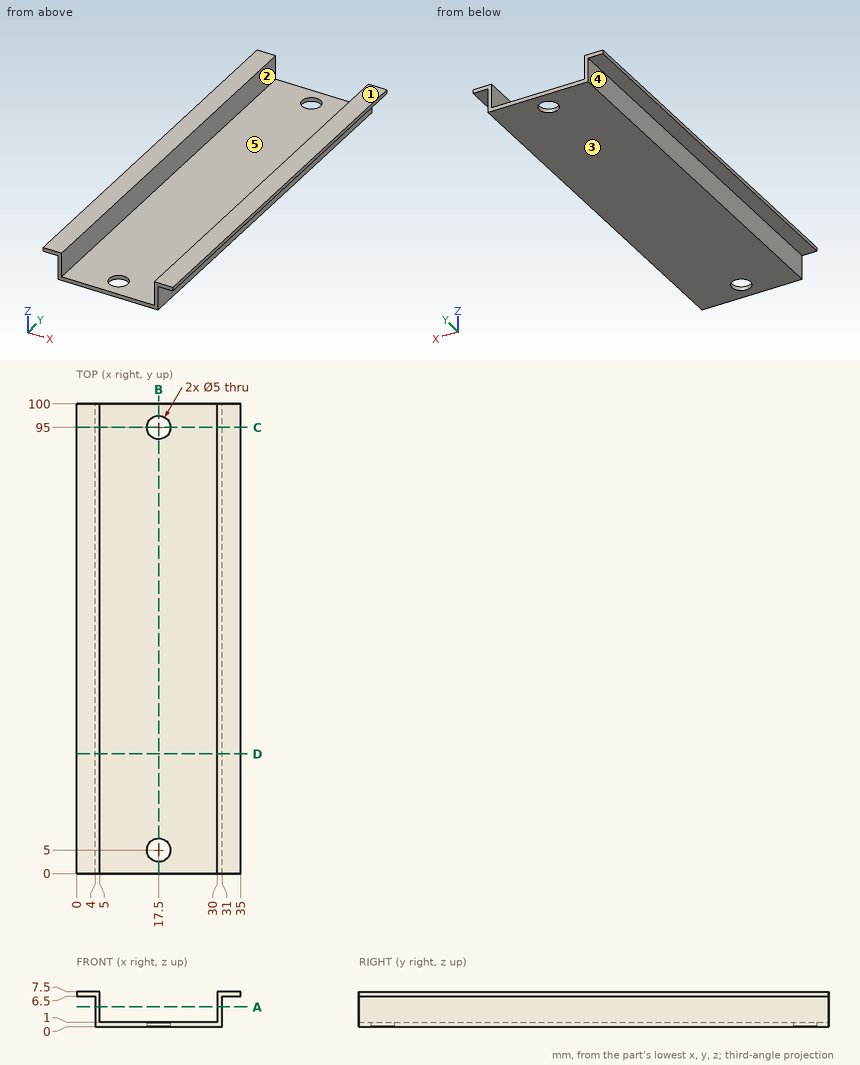
Verification items for this drawing (mm, ordinates from the low corner). A direction names the side the tool comes from. Give positions to 0.01 mm unless a question says otherwise; leave off trailing zeros. Loops run counter-clockwise (first coordinate to the right, second up) from the corner with the lowest first, then second, coordinate; pieces in that order, holes last.
1. Cross-section at B-B on x = 17.5. Record the cut outline in (y, z).
Derived:
outline: (0, 0) - (2.5, 0) - (2.5, 1) - (0, 1) - close; (7.5, 0) - (92.5, 0) - (92.5, 1) - (7.5, 1) - close; (97.5, 0) - (100, 0) - (100, 1) - (97.5, 1) - close
2. Material ranges on probe 1 along Y at (x, z) = (17.5, 0.45); probe 2 along X at (y, z) = (88.5, 2.5); probe 3 along X at (y, z) = (6, 7), recorded low to high.
Derived:
probe 1: y = 0 to 2.5, 7.5 to 92.5, 97.5 to 100
probe 2: x = 4 to 5, 30 to 31
probe 3: x = 0 to 5, 30 to 35
3. Cross-section at D-D on y = 25.5. Record the cut outline in (x, z).
Derived:
outline: (0, 6.5) - (4, 6.5) - (4, 0) - (31, 0) - (31, 6.5) - (35, 6.5) - (35, 7.5) - (30, 7.5) - (30, 1) - (5, 1) - (5, 7.5) - (0, 7.5) - close
4. Release check for a two-part mould opening along X. For the marked faces 3, 4 and 5 record: +X half, -X half, draft (parallel to the pull), parting line (faces both ways), or undercut.
Derived:
face 3: draft
face 4: -X half
face 5: undercut
5. Cross-section at C-C on y = 95. Record the cut outline in (x, z).
Derived:
outline: (0, 6.5) - (4, 6.5) - (4, 0) - (15, 0) - (15, 1) - (5, 1) - (5, 7.5) - (0, 7.5) - close; (20, 0) - (31, 0) - (31, 6.5) - (35, 6.5) - (35, 7.5) - (30, 7.5) - (30, 1) - (20, 1) - close
6. Cross-section at A-A on z = 4.25. Record the cut outline in (x, y), and give its area (3 significant figures).
Derived:
outline: (4, 0) - (5, 0) - (5, 100) - (4, 100) - close; (30, 0) - (31, 0) - (31, 100) - (30, 100) - close
area: 200 mm2
7. Tool access check on the marked faces 1 and 2. Record the directions out of +Z, -Z, +X, -X, +Y, -Y that give a thin tool (end or side, any length) a straight path to the whole face; none if there is none.
Derived:
face 1: +Z, +X, -X, +Y, -Y
face 2: +Z, +Y, -Y
8. Go/stop test with flat-tipped pins: P1, Ø8, axis at x = 17.5, y = 19, coming from the +Z side; P2, Ø3, axis at y = 27.5, z = 3, coming from the -X side; P3, Ø3, axis at x = 2, y = 36, coming from the -Z side; P4, Ø4, axis at x = 17.5, y = 95, coming from the +Z side. Record where each tip stops, or that it passes through.
Derived:
P1: stops at z = 1
P2: stops at x = 4
P3: stops at z = 6.5
P4: passes through
